Check sheet for the modelled part. Datum: model origin and axes. Units: mm. Give positions to 0.01 mm unless a question says otherwise; leave off trailing zeros. Order: outer loops, then holes, each group sorted by start corner. A loop starts at its lowest first (then second) coordinate and runs counter-clockwise, first axis right, second up.
Solid Edge part; units mm, degrees
sketch "Sketch1" plane through (0, 0, 0) normal (1, 0, 0) x (0, 1, 0)
  line L0 (95.5215, -16.3706) -> (87.5215, -16.3706)
  line L1 (87.5215, -16.3706) -> (87.5215, -57.067)
  line L2 (87.5215, -57.067) -> (95.5215, -57.067)
  line L3 (95.5215, -57.067) -> (95.5215, -16.3706)
  circle A0 centre (90.8215, -32.0096) radius 1.7
  dimension "D1" = 95.5215
extrude "Protrusion1" add sketch "Sketch1" against normal blind 1
sketch "Sketch2" plane through (0, 91.5215, -36.7188) normal (1, 0, 0) x (0, 0, 1)
  line L0 (-5.4908, -4) -> (-25.4908, 16)
  line L1 (-25.4908, 16) -> (-24.9247, -9.9187)
  line L2 (-24.9247, -9.9187) -> (-5.4908, -4)
  line L3 (14.2188, -4) -> (34.2188, 16)
  line L4 (34.2188, 16) -> (29.5856, -11.0555)
  line L5 (29.5856, -11.0555) -> (14.2188, -4)
extrude "ExtrudedCutout_1" cut sketch "Sketch2" against normal blind 36
(1) Cross-section at D-D on y = 93. Enter the section's corners in (x, z).
Response values:
outline: (-1, -44.73) - (0, -44.73) - (0, -19.98) - (-1, -19.98) - close
(2) Release check for a two-part mould opening along Z. For faces 1 (the face through (-0.493, 89.123, -31.935)), 2 (the face through (-0.49, 91.58, -46.15)), 3 (the face through (-0.5, 88.5, -16.371)), 4 (the face through (-0.5, 95.522, -32.5)) record: released by +Z, released by -Z, zero draft, split by the parting line, or undercut.
Response values:
face 1: undercut
face 2: released by -Z
face 3: released by +Z
face 4: zero draft
(3) Cross-section at C-C on x = -0.45. Enter the section's corners in (y, z).
Response values:
outline: (87.52, -50.21) - (95.52, -42.21) - (95.52, -22.5) - (89.39, -16.37) - (87.52, -16.37) - close; hole circle Ø3.4 at (90.82, -32.01)
(4) Material ranges on L1, parallel to Y at x = -0.9, z = -31; L2, parallel to Z at x = -0.7, y = 91.25; L3, parallel to Y at x = -0.55, z = -32.5, recorded low to high.
Response values:
L1: y = 87.52 to 89.45, 92.19 to 95.52
L2: z = -46.48 to -33.65, -30.36 to -18.23
L3: y = 87.52 to 89.19, 92.45 to 95.52
(5) Cross-section at B-B on y = 90.75. Enter the section's corners in (x, z), then the cut area to 3 significant figures.
Response values:
outline: (-1, -46.98) - (0, -46.98) - (0, -33.71) - (-1, -33.71) - close; (-1, -30.31) - (0, -30.31) - (0, -17.73) - (-1, -17.73) - close
area: 25.9 mm2
(6) Cross-section at A-A on z = -33. Enter the section's corners in (x, y), then the cut area to 3 significant figures.
Response values:
outline: (-1, 87.52) - (0, 87.52) - (0, 89.44) - (-1, 89.44) - close; (-1, 92.2) - (0, 92.2) - (0, 95.52) - (-1, 95.52) - close
area: 5.24 mm2
